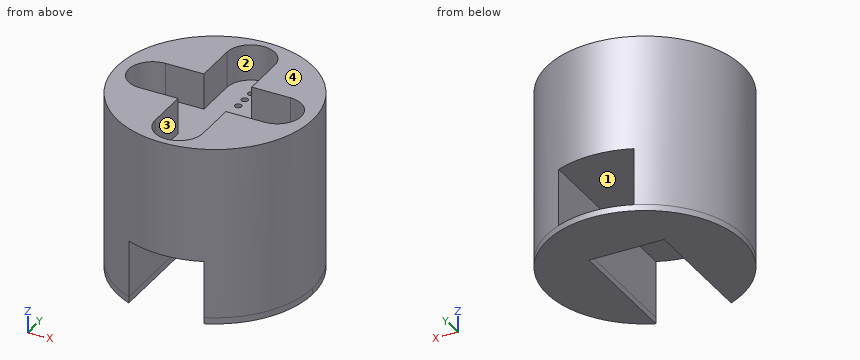
from build123d import *

# Parameters (mm, degrees)
SKETCH1_R           = 23.5
BOSS_EXTRUDE1_DEPTH = 41.47
SKETCH5_W           = 18.1
SKETCH5_H           = 47
CUT_EXTRUDE1_DEPTH  = 13.8
SKETCH6_R           = 23.5
BOSS_EXTRUDE2_DEPTH = 1.5
CUT_EXTRUDE5_DEPTH  = 1.5
CUT_EXTRUDE10_DEPTH = 8.67
SKETCH14_R          = 0.8
SKETCH14_R_2        = 0.668140713
CUT_EXTRUDE12_DEPTH = 1


with BuildPart() as part:
    # Sketch1 → Boss-Extrude1 (new body)
    with BuildSketch(Plane.XY):
        Circle(SKETCH1_R)
    extrude(amount=BOSS_EXTRUDE1_DEPTH)

    # Sketch5 → Cut-Extrude1 (cut)
    with BuildSketch(Plane(origin=(0, 0, 0), x_dir=(-1, 0, 0), z_dir=(0, 0, -1))):
        Rectangle(SKETCH5_W, SKETCH5_H)
    extrude(amount=-CUT_EXTRUDE1_DEPTH, mode=Mode.SUBTRACT)

    # Sketch6 → Boss-Extrude2 (add)
    with BuildSketch(Plane.XY):
        Circle(SKETCH6_R)
    extrude(amount=-BOSS_EXTRUDE2_DEPTH)

    # Sketch8 → Cut-Extrude5 (cut)
    with BuildSketch(Plane(origin=(0, 0, -1.5), x_dir=(-1, 0, 0), z_dir=(0, 0, -1))):
        with BuildLine():
            Line((-9.05, 8.2), (9.05, 8.2))
            Line((9.05, 8.2), (9.05, -21.687496398))
            ThreePointArc((9.05, -21.687496398), (0, -23.5), (-9.05, -21.687496398))
            Line((-9.05, -21.687496398), (-9.05, 8.2))
        make_face()
    extrude(amount=-CUT_EXTRUDE5_DEPTH, mode=Mode.SUBTRACT)

    # Sketch9 → Cut-Extrude10 (cut)
    with BuildSketch(Plane.XY.offset(41.47)):
        with BuildLine():
            Line((-5.775203881, 16), (-5.775203881, 5.75))
            Line((-5.775203881, 5.75), (-15, 5.75))
            ThreePointArc((-15, 5.75), (-20.75, 0), (-15, -5.75))
            Line((-15, -5.75), (-5.775203881, -5.75))
            Line((-5.775203881, -5.75), (-5.775203881, -16))
            ThreePointArc((-5.775203881, -16), (-0.025205722, -21.749998159), (5.724792437, -16))
            Line((5.724792437, -16), (5.724792437, -5.75))
            Line((5.724792437, -5.75), (15, -5.75))
            ThreePointArc((15, -5.75), (20.75, 0), (15, 5.75))
            Line((15, 5.75), (5.724792437, 5.75))
            Line((5.724792437, 5.75), (5.724792437, 16))
            ThreePointArc((5.724792437, 16), (-0.025205722, 21.749998159), (-5.775203881, 16))
        make_face()
    extrude(amount=-CUT_EXTRUDE10_DEPTH, mode=Mode.SUBTRACT)

    # Sketch14 → Cut-Extrude12 (cut)
    with BuildSketch(Plane.XY.offset(32.8)):
        with Locations((0, 18.949998159)):
            Circle(SKETCH14_R)
        with Locations((0, 18.949998159)):
            Circle(SKETCH14_R_2, mode=Mode.SUBTRACT)
        with Locations((0, 10.399998159)):
            Circle(SKETCH14_R)
        with Locations((0, 13.249998159)):
            Circle(SKETCH14_R)
        with Locations((0, 16.099998159)):
            Circle(SKETCH14_R)
        with Locations((0, -10.399998159)):
            Circle(SKETCH14_R)
        with Locations((0, -13.249998159)):
            Circle(SKETCH14_R)
        with Locations((0, -16.099998159)):
            Circle(SKETCH14_R)
        with Locations((0, -18.949998159)):
            Circle(SKETCH14_R)
        with Locations((12.25, 0)):
            Circle(SKETCH14_R)
        with Locations((15.1, 0)):
            Circle(SKETCH14_R)
        with Locations((17.95, 0)):
            Circle(SKETCH14_R)
        with Locations((-12.25, 0)):
            Circle(SKETCH14_R)
        with Locations((-15.1, 0)):
            Circle(SKETCH14_R)
        with Locations((-17.95, 0)):
            Circle(SKETCH14_R)
    extrude(amount=-CUT_EXTRUDE12_DEPTH, mode=Mode.SUBTRACT)


solid = part.part
Source: CAD feature listing. Evaluate the final solid. Frame: model axes, mm. Face numbers are marked on the shaded views. A direction names the side the tool comes from. Round coordinates to 2 decimals unless told otherwise and drop trailing zeros. Loops run counter-clockwise (first coordinate to the right, second up) from the corner with the lowest first, then second, coordinate; pieces in that order, holes last. Notation, with made-up numbers: (-24.5, 9.25) - (-3.5, 9.25) arc R7 cw to (-3.5, 21.25) - close; hole circle Ø7 at (-38.5, -31). An arc over 180 degrees is marked (long way). Write item = value, one per line. Start each with the question number.
Item 1: Material intervals for line 1 (X direction, y = 11, z = 4); line 2 (Z direction, x = 4.5, y = 9); line 3 (Y direction, x = 11, z = 22), sorted ascending.
Item 2: Section query A-A on z = 12. Output: boundary loops of the cut face in (x, y).
Item 3: Section query C-C on y = 7. Output: boundary loops of the cut face in (x, z), plus the area to 3 significant figures.
Item 4: Section query B-B on x = 1.5. Output: boundary loops of the cut face in (y, z), plus the area to 3 significant figures.
Item 5: First-contact query: pin 1 Ø2 at (x, y) = (0, -13.25) entering from -Z; pin 2 Ø2.5 at (x, y) = (0, 16.1) entering from +Z; pin 3 Ø7 at (x, z) = (-9, 36.5) entering from -Y; pin 4 Ø12 at (y, z) = (-5.5, 3.5) entering from +X. Flat tips, straight axial feed; report the tip coordinate or a pass-through.
Item 6: Section query D-D on x = 12.25. Output: boundary loops of the cut face in (y, z), plus the area to 3 significant figures.
Item 7: Mould query, pull axis Y, two halves, no side actions, for the marked faces 1 and 2. Classes: released by +Y, released by -Y, zero draft, split by the parting line, or undercut.
Item 8: Reachability of the marked faces 3 and 4 from +Z, -Z, +X, -X, +Y, -Y: full face, straight path, thin tool, end or side. Return the list, or none.
Results list:
q1.line_1 = -20.77 to -9.05, 9.05 to 20.77
q1.line_2 = -1.5 to 0, 13.8 to 32.8
q1.line_3 = -20.77 to 20.77
q2.outline = (-9.05, -21.69) - (-9.05, 21.69) arc R23.5 ccw to start; (9.05, -21.69) arc R23.5 ccw to (9.05, 21.69) - close
q3.outline = (-22.43, -1.5) - (-9.05, -1.5) - (-9.05, 13.8) - (9.05, 13.8) - (9.05, -1.5) - (22.43, -1.5) - (22.43, 41.47) - (5.72, 41.47) - (5.72, 32.8) - (-5.78, 32.8) - (-5.78, 41.47) - (-22.43, 41.47) - close
q3.area = 1,550 mm²
q4.outline = (-23.45, 13.8) - (23.45, 13.8) - (23.45, 41.47) - (21.54, 41.47) - (21.54, 32.8) - (-21.54, 32.8) - (-21.54, 41.47) - (-23.45, 41.47) - close; (8.2, -1.5) - (23.45, -1.5) - (23.45, 0) - (8.2, 0) - close
q4.area = 947 mm²
q5.pin_1 = 13.8
q5.pin_2 = 32.8
q5.pin_3 = -22.85
q5.pin_4 = 23.5
q6.outline = (-20.05, -1.5) - (20.05, -1.5) - (20.05, 41.47) - (5.75, 41.47) - (5.75, 32.8) - (0.8, 32.8) - (0.8, 31.8) - (-0.8, 31.8) - (-0.8, 32.8) - (-5.75, 32.8) - (-5.75, 41.47) - (-20.05, 41.47) - close
q6.area = 1,620 mm²
q7.face_1 = zero draft
q7.face_2 = undercut
q8.face_3 = +Z
q8.face_4 = +Z, +X, -X, +Y, -Y
